Design review of the part built by this model. Coordinates are the model's own, in mm. Face numbers are marked on the shaded views. A direction names the side the tool comes from. Coordinates: 2 decimals unless noted, no trailing zeros. Write each loop counter-clockwise with the first axis right and the second up, starting at its lowest first coordinate (ties: lowest second). Pieces come first, ordered by that corner, then holes.
Q1. Take a section at A-A, the plane z = -25.5. Write out the cut boundary in (x, y).
Q2. For the marked faces 1 and 2, list the 3-axis set-ups (+Z, -Z, +X, -X, +Y, -Y) from which the entire face can be reached by the end or side of a thin tool; tool diameter is ignored.
Q3. Take a section at C-C, the plane x = 34. Write out the cut boundary in (y, z).
Q4. Take a section at D-D, the plane y = 8. Write out the cut boundary in (x, z).
Q5. For pin 1 Ø5 at (y, z) = (11, -31.5) entering from +X; pin 2 Ø9 at (x, z) = (71.76, -25.93) entering from +Y; pin 3 Ø6.5 at (x, z) = (71.52, -69.74) entering from -Y, all flat-tipped, find the tip position at first contact; note any pin that passes through.
Q6. For L1, parallel to X at y = 3.5, z = -79; L2, parallel to Y at x = 95.5, z = -85.5, list the stretches that pass through material, from the lowest coordinate up.
Q7. Take a section at B-B, the plane z = -52. Write out the cut boundary in (x, y), plus the area to 3 significant figures.
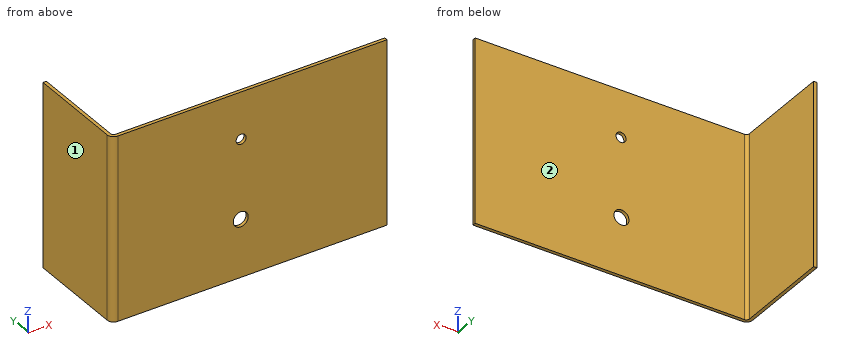
from build123d import *

# Parameters (mm, degrees)
SKETCH1_W                    = 152.4
SKETCH1_H                    = 101.6
BASE_FLANGE1_DEPTH           = 1.8542
EDGE_FLANGE1_STRIP_W         = 10.7442
EDGE_FLANGE1_STRIP_H         = 1.8542
EDGE_FLANGE1_STRIP_CUT_DEPTH = 101.6
EDGE_FLANGE1_DEPTH           = 101.6
SKETCH14_R                   = 2.7813
TAP_1_4_20_HOLE1_DEPTH       = 2.54
SKETCH15_R                   = 4.1413765
TAPPED_3_8_16_HOLE2_DEPTH    = 2.54


# Sheet-metal steps are written as plain solids
with BuildPart() as part:
    # Sketch1 → Base-Flange1 (new body)
    with BuildSketch(Plane(origin=(0, 0, 0), x_dir=(1, 0, 0), z_dir=(0, 1, 0))):
        with Locations((76.2, 50.8)):
            Rectangle(SKETCH1_W, SKETCH1_H)
    extrude(amount=-BASE_FLANGE1_DEPTH)

    # Edge-Flange1 strip (across the edge) → Edge-Flange1 strip cut (cut)
    with BuildSketch(Plane.XY.offset(-101.6)):
        with Locations((-1.8542, -0.9271)):
            Rectangle(EDGE_FLANGE1_STRIP_W, EDGE_FLANGE1_STRIP_H)
    extrude(amount=EDGE_FLANGE1_STRIP_CUT_DEPTH, mode=Mode.SUBTRACT)

    # Edge-Flange1 section (across the edge) → Edge-Flange1 (add)
    with BuildSketch(Plane.XY.offset(-101.6)):
        with BuildLine():
            Line((0, 1.6637), (0, 55.3339))
            Line((0, 55.3339), (1.8542, 55.3339))
            Line((1.8542, 55.3339), (1.8542, 1.6637))
            ThreePointArc((1.8542, 1.6637), (2.341486448, 0.487286448), (3.5179, 0))
            Line((3.5179, 0), (3.5179, -1.8542))
            ThreePointArc((3.5179, -1.8542), (1.030369054, -0.823830946), (0, 1.6637))
        make_face()
    extrude(amount=EDGE_FLANGE1_DEPTH)

    # Sketch14 → TAP 1/4-20 Hole1 (cut)
    with BuildSketch(Plane(origin=(0, 0, 0), x_dir=(1, 0, 0), z_dir=(0, 1, 0))):
        with Locations(Location((71.763910774, 25.92775269, 0), (0, 0, 270))):
            Circle(SKETCH14_R)
    extrude(amount=-TAP_1_4_20_HOLE1_DEPTH, mode=Mode.SUBTRACT)

    # Sketch15 → TAPPED 3/8-16 Hole2 (cut)
    with BuildSketch(Plane(origin=(0, 0, 0), x_dir=(1, 0, 0), z_dir=(0, 1, 0))):
        with Locations(Location((71.515516592, 69.738450307, 0), (0, 0, 270))):
            Circle(SKETCH15_R)
    extrude(amount=-TAPPED_3_8_16_HOLE2_DEPTH, mode=Mode.SUBTRACT)


solid = part.part
Responses:
1. outline: (0, 1.66) arc R3.52 ccw to (3.52, -1.85) - (69.02, -1.85) - (69.02, 0) - (3.52, 0) arc R1.66 cw to (1.85, 1.66) - (1.85, 55.33) - (0, 55.33) - close; (74.51, -1.85) - (152.4, -1.85) - (152.4, 0) - (74.51, 0) - close
2. face 1: +Z, -Z, -X, +Y, -Y
2. face 2: +Z, -Z, +X, +Y
3. outline: (-1.85, -101.6) - (0, -101.6) - (0, 0) - (-1.85, 0) - close
4. outline: (0, -101.6) - (1.85, -101.6) - (1.85, 0) - (0, 0) - close
5. pin 1: stops at x = 1.85
5. pin 2: stops at y = 0
5. pin 3: passes through
6. L1: x = 0 to 1.85
6. L2: y = -1.85 to 0
7. outline: (0, 1.66) arc R3.52 ccw to (3.52, -1.85) - (152.4, -1.85) - (152.4, 0) - (3.52, 0) arc R1.66 cw to (1.85, 1.66) - (1.85, 55.33) - (0, 55.33) - close
7. area: 383 mm2
